Part model, mm, in its own coordinate system. Coordinates: 2 decimals unless noted, no trailing zeros. Write each loop counter-clockwise with the first axis right and the second up, starting at its lowest first coordinate (ties: lowest second). Pieces come first, ordered by that corner, then holes. Notation, with made-up numbers: (47, 85.25) -> (64, 85.25) arc R21 cw to (64, 122.25) -> close; hole circle Ø9 at (70.25, 46.25). An arc over 180 degrees is marked (long way). One line per question, with ' | ' between items. Start each with the question number.
Item 1: Probe probe 1 along X at (y, z) = (43.25, 19); probe 2 along Z at (x, y) = (7, 43.5); probe 3 along Z at (x, y) = (3.5, 41.25). List the from-to ranges inside material, lowest first. Write a range as [from, to].
Item 2: Saw through at B-B (z = 1.5). List the corners of the cut face in (x, y).
Item 3: Saw through at A-A (y = 39.5). List the corners of the cut face in (x, z), and give its area (3 significant figures).
Item 4: Pin check, flat tip, straight feed: pin 1 (1.5 mm diameter, centred on x = 16.5, y = 39.5, fed in from +Z). Stop position of the tip, or through.
Item 5: Saw through at C-C (x = 5). List the corners of the cut face in (y, z).
from build123d import *

# Parameters (mm, degrees)
CIRCLE_AS_DRAWN_R                       = 11.25
EXTRUDE002_DEPTH                        = 13
EXTRUDE002_ONTO_CIRCLE_ROLL_ANGLE       = 90
EXTRUDE002_ONTO_CIRCLE_PLACEMENT_ANGLE  = 180
RECTANGLE004_AS_DRAWN_W                 = 17.799999
RECTANGLE004_AS_DRAWN_H                 = 22.34914
EXTRUDE008_DEPTH                        = 13
EXTRUDE008_ONTO_RECTANGLE004_ROLL_ANGLE = 90


with BuildPart() as caixamotor:
    # Circle as drawn → Extrude002 (new)
    with BuildSketch(Plane.XY):
        Circle(CIRCLE_AS_DRAWN_R)
    extrude(amount=EXTRUDE002_DEPTH)


with BuildPart() as caixamotor_1:
    # Extrude002 onto Circle roll: moved
    add(caixamotor.part.rotate(Axis((0, 0, 0), (1, 0, 0)), EXTRUDE002_ONTO_CIRCLE_ROLL_ANGLE))


with BuildPart() as caixamotor_2:
    # Extrude002 onto Circle placement: moved
    add(caixamotor_1.part.moved(Location((9.4, 37, 11.25))).rotate(Axis((9.4, 37, 11.25), (0, 0, 1)), EXTRUDE002_ONTO_CIRCLE_PLACEMENT_ANGLE))


with BuildPart() as booleancaixamotor:
    # Rectangle004 as drawn → Extrude008 (new)
    with BuildSketch(Plane.XY):
        with Locations((8.899999, -11.17457)):
            Rectangle(RECTANGLE004_AS_DRAWN_W, RECTANGLE004_AS_DRAWN_H)
    extrude(amount=-EXTRUDE008_DEPTH)


with BuildPart() as booleancaixamotor_1:
    # Extrude008 onto Rectangle004 roll: moved
    add(booleancaixamotor.part.rotate(Axis((0, 0, 0), (1, 0, 0)), EXTRUDE008_ONTO_RECTANGLE004_ROLL_ANGLE))


with BuildPart() as booleancaixamotor_2:
    # Extrude008 onto Rectangle004 placement: moved
    add(booleancaixamotor_1.part.moved(Location((0.516884, 1.09014, 22.397291))))


with BuildPart() as booleancaixamotor_3:
    # Extrude008 placement: moved
    add(booleancaixamotor_2.part.moved(Location((0, 36, 0))))

    # Common: intersect CaixaMotor
    add(caixamotor_2.part, mode=Mode.INTERSECT)


with BuildPart() as booleancaixamotor_4:
    # Common placement: moved
    add(booleancaixamotor_3.part.moved(Location((0.5, -0.1, 0))))


solid = booleancaixamotor_4.part
From the geometry:
1) probe 1: [1.75, 18.05] | probe 2: [0.38, 22.12] | probe 3: [2, 20.5]
2) outline: (4.29, 36.99) -> (15.51, 36.99) -> (15.51, 49.9) -> (4.29, 49.9) -> close
3) outline: (1.02, 4.35) arc R11.25 ccw to (8.86, 0.05) -> (10.94, 0.05) arc R11.25 ccw to (18.82, 4.39) -> (18.82, 18.11) arc R11.25 ccw to (11.42, 22.4) -> (8.38, 22.4) arc R11.25 ccw to (1.02, 18.15) -> close | area: 353 mm2
4) pin 1: z = 20.86
5) outline: (36.99, 1.12) -> (49.9, 1.12) -> (49.9, 21.38) -> (36.99, 21.38) -> close
